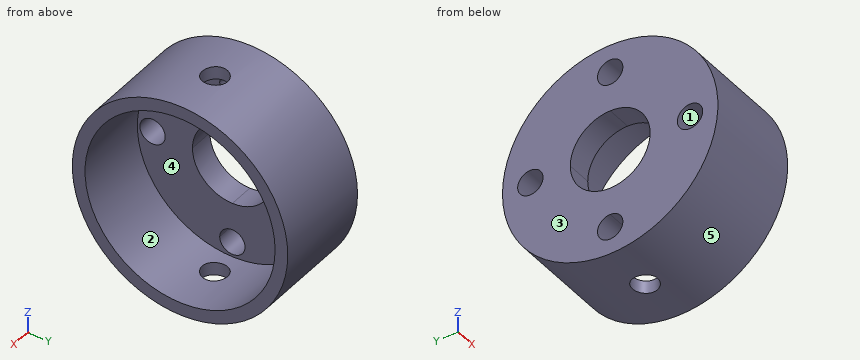
```python
from build123d import *

# Parameters (mm, degrees)
F0_R     = 10.795
F0_R_2   = 9.525
F1_DEPTH = 10.16
F2_DEPTH = 2.54
F4_DEPTH = 25.4
F5_DEPTH = 25.4
F6_R     = 1.27
F7_DEPTH = 25.4


with BuildPart() as f1:
    # F0 (on Right) → F1 (new body)
    with BuildSketch(Plane.YZ):
        Circle(F0_R)
        Circle(F0_R_2, mode=Mode.SUBTRACT)
    extrude(amount=F1_DEPTH)

    # F0 (on Right) → F2 (join)
    with BuildSketch(Plane.YZ):
        Circle(F0_R_2)
    extrude(amount=F2_DEPTH)

    # F3 (on Top) → F4 (cut)
    with BuildSketch(Plane.XY):
        with BuildLine():
            ThreePointArc((3.81, 0), (5.08, -1.27), (6.35, 0))
            ThreePointArc((6.35, 0), (5.08, 1.27), (3.81, 0))
        make_face()
    extrude(amount=-F4_DEPTH, mode=Mode.SUBTRACT)

    # F3 (on Top) → F5 (cut)
    with BuildSketch(Plane.XY):
        with BuildLine():
            ThreePointArc((3.81, 0), (5.08, -1.27), (6.35, 0))
            ThreePointArc((6.35, 0), (5.08, 1.27), (3.81, 0))
        make_face()
    extrude(amount=F5_DEPTH, mode=Mode.SUBTRACT)

    # F6 (on face) → F7 (cut)
    with BuildSketch(Plane(origin=(0, 0, 0), x_dir=(0, -1, 0), z_dir=(-1, 0, 0))):
        with BuildLine():
            ThreePointArc((1.27, 8.001), (-0.8980256121, 8.8990256121), (0, 6.731))
            ThreePointArc((0, 6.731), (0.8980256121, 7.1029743879), (1.27, 8.001))
        make_face()
        with Locations((-8.001, 0)):
            Circle(F6_R)
        with BuildLine():
            ThreePointArc((1.27, -8.001), (0.8980256121, -7.1029743879), (0, -6.731))
            ThreePointArc((0, -6.731), (-0.8980256121, -8.8990256121), (1.27, -8.001))
        make_face()
        with BuildLine():
            ThreePointArc((9.271, 0), (8.001, 1.27), (6.731, 0))
            ThreePointArc((6.731, 0), (8.001, -1.27), (9.271, 0))
        make_face()
        with BuildLine():
            Line((0, 0), (4.0005, 0))
            ThreePointArc((4.0005, 0), (2.8287806781, 2.8287806781), (0, 4.0005))
            Line((0, 4.0005), (0, 0))
        make_face()
        with BuildLine():
            Line((0, 0), (0, 4.0005))
            ThreePointArc((0, 4.0005), (-2.8287806781, 2.8287806781), (-4.0005, 0))
            Line((-4.0005, 0), (0, 0))
        make_face()
        with BuildLine():
            ThreePointArc((-4.0005, 0), (-2.8287806781, -2.8287806781), (0, -4.0005))
            Line((0, -4.0005), (0, 0))
            Line((0, 0), (-4.0005, 0))
        make_face()
        with BuildLine():
            ThreePointArc((0, -4.0005), (2.8287806781, -2.8287806781), (4.0005, 0))
            Line((4.0005, 0), (0, 0))
            Line((0, 0), (0, -4.0005))
        make_face()
    extrude(amount=-F7_DEPTH, mode=Mode.SUBTRACT)


solid = f1.part
```
Verification items for the finished model (mm, model axes). Face numbers are marked on the shaded views. A direction names the side the tool comes from. Coordinates: 2 decimals unless noted, no trailing zeros. Write each loop counter-clockwise with the first axis right and the second up, starting at its lowest first coordinate (ties: lowest second). Pieces come first, ordered by that corner, then holes. Notation, with made-up numbers: M -17,46 L 28,46 A18 ccw 28,79 Z; hole C 88.5,-28.5 d5. An arc over 180 degrees is marked long. Answer as a JSON object with one key per item and string values. Group by question number.
(1) Cross-section at B-B, the plane x = 5.08. Record the cut outline in (y, z) (3 decimals), and give its area (3 significant figures).
(2) Release check for a two-part mould opening along Y. For the marked faces 3, 4 and 5 record: +Y half, -Y half, draft (parallel to the pull), parting line (faces both ways), or undercut.
(3) Cross-section at C-C, the plane z = 1. Record the cut outline in (x, y), and give its area (3 significant figures).
(4) Cross-section at A-A, the plane x = 1.75. Record the cut outline in (y, z) (1 decimal).
(5) Material ranges on line 1 (Z direction, x = 7.5, y = 0) (3 decimals); line 2 (X direction, y = -7.25, z = -5); line 3 (X direction, y = 0, z = -10.5), recorded low to high.
(6) Tool access check on the marked faces 1 and 2. Record the directions out of +Z, -Z, +X, -X, +Y, -Y that give a thin tool (end or side, any length) a straight path to the whole face; none if there is none.
(7) Gauge pin test, flat ends, axial feed: pin 1 (5.5 mm diameter, centred on y = -4, z = -1, fed in from +X); pin 2 (1 mm diameter, centred on x = 1.5, z = -2, fed in from -Y); pin 3 (2 mm diameter, centred on x = 8, y = -8.5, fed in from -Z). Record the tip position at first contact, or that the pin passes through.
(8) Cross-section at D-D, the plane y = -4.5. Record the cut outline in (x, z).
Reply:
{
 "1": {"outline": "M -1.27,-10.72 L -1.27,-9.44 A9.525 cw -1.27,9.44 L -1.27,10.72 A10.795 ccw Z; M 1.27,-10.72 A10.795 ccw 1.27,10.72 L 1.27,9.44 A9.525 cw 1.27,-9.44 Z", "area": "74.6 mm²"},
 "2": {"face 3": "draft", "face 4": "undercut", "face 5": "parting line"},
 "3": {"outline": "M 0,-10.75 L 10.16,-10.75 L 10.16,-9.47 L 2.54,-9.47 L 2.54,-8.78 L 0,-8.78 Z; M 0,-7.22 L 2.54,-7.22 L 2.54,-3.87 L 0,-3.87 Z; M 0,3.87 L 2.54,3.87 L 2.54,7.22 L 0,7.22 Z; M 0,8.78 L 2.54,8.78 L 2.54,9.47 L 10.16,9.47 L 10.16,10.75 L 0,10.75 Z", "area": "46.4 mm²"},
 "4": {"outline": "C 0,0 d21.6; hole C -8,0 d2.5; hole C 0,0 d8; hole C 0,-8 d2.5; hole C 0,8 d2.5; hole C 8,0 d2.5"},
 "5": {"line 1": "-10.795 to -9.525, 9.525 to 10.795", "line 2": "0 to 2.54", "line 3": "0 to 3.81, 6.35 to 10.16"},
 "6": {"face 1": "+X, -X", "face 2": "+X"},
 "7": {"pin 1": "x = 2.54", "pin 2": "y = -10.69", "pin 3": "z = -7.76"},
 "8": {"outline": "M 0,-9.81 L 10.16,-9.81 L 10.16,-8.39 L 2.54,-8.39 L 2.54,8.39 L 10.16,8.39 L 10.16,9.81 L 0,9.81 Z"}
}
